Answer from the drawing. Dimensions are ordinates in mm from the lowest x, y and z of the part. A direction names the side the tool comes from. Give positions to 0.01 mm unless a question says otherwise; leave off trailing zeros. Order: outer loops, then holes, each group sorted by start corner. A loop starts at its lowest first (then second) coordinate and runs counter-clockwise, first axis right, second up. Notation, with made-up numbers: (-16.5, 22) - (29.5, 22) arc R27 cw to (29.5, 55) - close; hole circle Ø5 at (-8, 53). An arc over 180 degrees is marked (long way). Write each question's results on one line, items separated by ' | '.
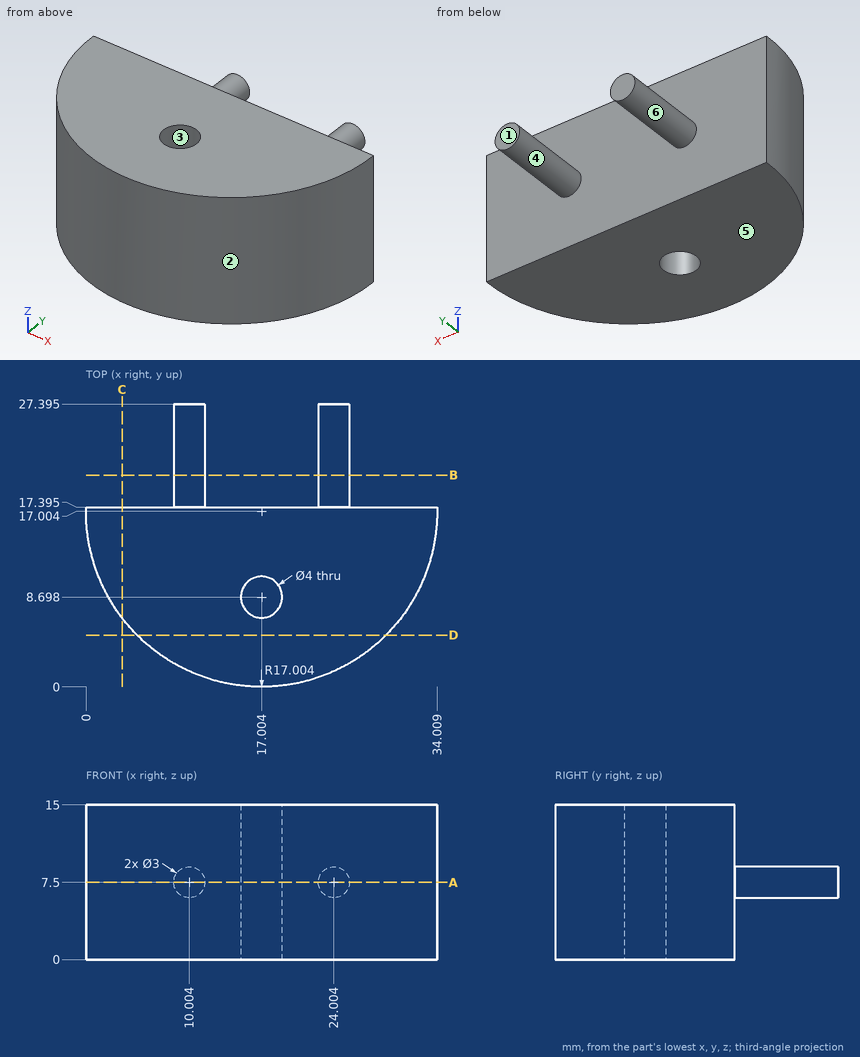
(1) Section B-B (y = 20.5) is taken. Give the vertices of the cut face in (x, z) (1 decimal).
Conclusion:
outline: circle Ø3 at (10, 7.5); circle Ø3 at (24, 7.5)
(2) The mould has two halves that part along X. Classify the marked faces 1, 2, 3 and 4: pulls with the +X half, pulls with the -X half, needs draft (parallel to the pull), parting line crosses it, or undercut.
Conclusion:
face 1: needs draft | face 2: parting line crosses it | face 3: undercut | face 4: undercut
(3) Section A-A (z = 7.5) is taken. Give the vertices of the cut face in (x, y) (1 decimal).
Conclusion:
outline: (0, 17.4) arc R17 ccw (long way) to (34, 17.4) - (25.5, 17.4) - (25.5, 27.4) - (22.5, 27.4) - (22.5, 17.4) - (11.5, 17.4) - (11.5, 27.4) - (8.5, 27.4) - (8.5, 17.4) - close; hole circle Ø4 at (17, 8.7)
(4) For the marked faces 5 and 6, determine the directions among +Z, -Z, +X, -X, +Y, -Y from which every point of the face is accessible in a straight line to the end or side of a thin tool.
Conclusion:
face 5: -Z, +X, -X, +Y, -Y | face 6: +Y
(5) Each of these flat-tipped pins is pushed along its axis until it touches: pin 1 (8 mm diameter, centred on y = 21.5, z = 11.5, fed in from +X) (1 decimal); pin 2 (2 mm diameter, centred on x = 23, z = 5, fed in from +Y) (1 decimal); pin 3 (6 mm diameter, centred on y = 3, z = 13, fed in from +X); pin 4 (4 mm diameter, centred on y = 15.5, z = 8, fed in from +X). Where does it stop, or does it pass through?
Conclusion:
pin 1: x = 25.5 | pin 2: y = 17.4 | pin 3: x = 29.97 | pin 4: x = 34.01
(6) Section D-D (y = 5) is taken. Give the vertices of the cut face in (x, z).
Conclusion:
outline: (4.96, 0) - (29.05, 0) - (29.05, 15) - (4.96, 15) - close
(7) Consider probe 1 along Y at (x, z) = (17, 1) (1 decimal); probe 2 along X at (y, z) = (17, 5.5); probe 3 along X at (y, z) = (26, 8.5) (1 decimal). Determine where each line is inside the solid, lowest interval first. Write a range as [from, to].
Conclusion:
probe 1: [0, 6.7], [10.7, 17.4] | probe 2: [0, 34.01] | probe 3: [8.9, 11.1], [22.9, 25.1]
(8) Section C-C (x = 3.5) is taken. Give the vertices of the cut face in (y, z) (1 decimal).
Conclusion:
outline: (6.7, 0) - (17.4, 0) - (17.4, 15) - (6.7, 15) - close
